Here's how the part is built. I have some questions about the finished solid (model axes, mm). Face numbers are marked on the shaded views. A direction names the side the tool comes from. Coordinates: 2 decimals unless noted, no trailing zeros. Write each loop counter-clockwise with the first axis right and the second up, starting at its lowest first coordinate (ties: lowest second). Pieces come first, ordered by that corner, then holes.
(1) Please list where these lines run through material, in increasing order: probe 1 along X at (y, z) = (1.8, 101.6); probe 2 along X at (y, z) = (1.55, 127); probe 3 along Y at (x, z) = (-7.5, 73.5).
(2) Thinking about a two-plate mould opening in Z: for the marked faces 1 and 2, which applies, released by +Z, released by -Z, zero draft, split by the parting line, or undercut?
(3) Imagine slicing it at D-D, the plane z = 127. List the corners of the cut face in (x, y) for me, plus the area to 3 significant figures.
(4) Imagine slicing it at B-B, the plane z = 50.8. List the corners of the cut face in (x, y) for me, plus the area to 3 significant figures.
(5) For pin 1 Ø10 at (x, z) = (2, 153.5) entering from +Y; pin 2 Ø1.1 at (x, y) = (-7.5, 2) entering from -Z, each with a flat end and sliding along its axis, tell me the tip position at first contact or that it passes through.
(6) Which directions (+Z, -Z, +X, -X, +Y, -Y) give clear straight access to the entire face, cutting with the end or side of a thin tool? Please do the marked faces 3 and 4.
(7) Imagine slicing it at A-A, the plane x = -19.5. List the corners of the cut face in (y, z) for me, plus the area to 3 significant figures.
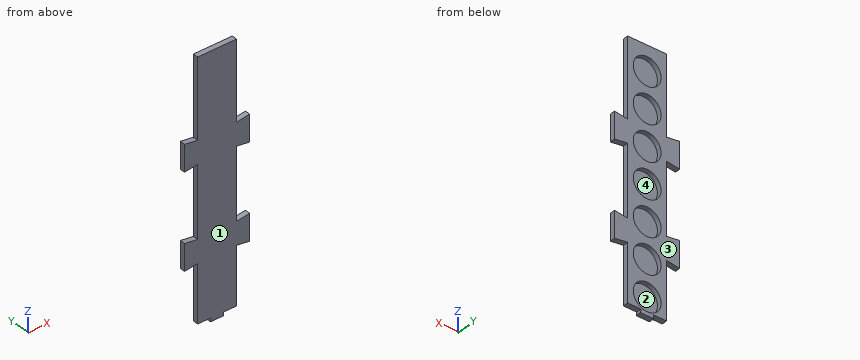
```python
from build123d import *

# Parameters (mm, degrees)
SKETCH1_W           = 27.94
SKETCH1_H           = 391.16
BOSS_EXTRUDE1_DEPTH = 3.81
SKETCH2_R           = 10
CUT_EXTRUDE1_DEPTH  = 3.21
BOSS_EXTRUDE2_DEPTH = 3.81
SKETCH7_W           = 46.80460671
SKETCH7_H           = 3.81
CUT_EXTRUDE2_DEPTH  = 210.82
BOSS_EXTRUDE4_DEPTH = 3.81


with BuildPart() as part:
    # Sketch1 → Boss-Extrude1 (new body)
    with BuildSketch(Plane(origin=(0, 0, 0), x_dir=(1, 0, 0), z_dir=(0, 1, 0))):
        Rectangle(SKETCH1_W, SKETCH1_H)
    extrude(amount=BOSS_EXTRUDE1_DEPTH)

    # Sketch2 → Cut-Extrude1 (cut)
    with BuildSketch(Plane(origin=(0, 3.81, 0), x_dir=(1, 0, 0), z_dir=(0, 1, 0))):
        with Locations(Location((0, 177.8, 0), (0, 0, 270))):
            Circle(SKETCH2_R)
        with Locations(Location((0, 152.4, 0), (0, 0, 270))):
            Circle(SKETCH2_R)
        with Locations(Location((0, 127, 0), (0, 0, 270))):
            Circle(SKETCH2_R)
        with Locations(Location((0, 101.6, 0), (0, 0, 270))):
            Circle(SKETCH2_R)
        with Locations(Location((0, 76.2, 0), (0, 0, 270))):
            Circle(SKETCH2_R)
        with Locations(Location((0, 50.8, 0), (0, 0, 270))):
            Circle(SKETCH2_R)
        with Locations(Location((0, 25.4, 0), (0, 0, 270))):
            Circle(SKETCH2_R)
        with Locations(Location((0, 0, 0), (0, 0, 270))):
            Circle(SKETCH2_R)
        with Locations(Location((0, -25.4, 0), (0, 0, 270))):
            Circle(SKETCH2_R)
        with Locations(Location((0, -50.8, 0), (0, 0, 270))):
            Circle(SKETCH2_R)
        with Locations(Location((0, -76.2, 0), (0, 0, 270))):
            Circle(SKETCH2_R)
        with Locations(Location((0, -101.6, 0), (0, 0, 270))):
            Circle(SKETCH2_R)
        with Locations(Location((0, -127, 0), (0, 0, 270))):
            Circle(SKETCH2_R)
        with Locations(Location((0, -152.4, 0), (0, 0, 270))):
            Circle(SKETCH2_R)
        with Locations(Location((0, -177.8, 0), (0, 0, 270))):
            Circle(SKETCH2_R)
    extrude(amount=-CUT_EXTRUDE1_DEPTH, mode=Mode.SUBTRACT)

    # Sketch4 → Boss-Extrude2 (add)
    with BuildSketch(Plane(origin=(0, 0, 0), x_dir=(1, 0, 0), z_dir=(0, 1, 0))):
        Polygon((23.402303355, -54.881033493), (13.97, -56.20665728), (13.97, -72.402209707), (23.402303355, -73.727833493), align=None)
        Polygon((23.402303355, 146.105623787), (13.97, 144.78), (13.97, 128.584447573), (23.402303355, 127.258823787), align=None)
        Polygon((-13.97, 128.584447573), (-13.97, 144.78), (-23.402303355, 146.105623787), (-23.402303355, 127.258823787), align=None)
        Polygon((23.402303355, 79.11007136), (13.97, 77.784447573), (13.97, 61.588895147), (23.402303355, 60.26327136), align=None)
        Polygon((23.402303355, 12.114518933), (13.97, 10.788895147), (13.97, -5.40665728), (23.402303355, -6.732281067), align=None)
        Polygon((-13.97, -5.40665728), (-13.97, 10.788895147), (-23.402303355, 12.114518933), (-23.402303355, -6.732281067), align=None)
        Polygon((-13.97, 61.588895147), (-13.97, 77.784447573), (-23.402303355, 79.11007136), (-23.402303355, 60.26327136), align=None)
        Polygon((23.402303355, -121.87658592), (13.97, -123.202209707), (13.97, -139.397762134), (23.402303355, -140.72338592), align=None)
        Polygon((-13.97, -139.397762134), (-13.97, -123.202209707), (-23.402303355, -121.87658592), (-23.402303355, -140.72338592), align=None)
        Polygon((-13.97, -72.402209707), (-13.97, -56.20665728), (-23.402303355, -54.881033493), (-23.402303355, -73.727833493), align=None)
    extrude(amount=BOSS_EXTRUDE2_DEPTH)

    # Sketch7 → Cut-Extrude2 (cut)
    with BuildSketch(Plane(origin=(0, 0, -195.58), x_dir=(-1, 0, 0), z_dir=(0, 0, -1))):
        with Locations((0, 1.905)):
            Rectangle(SKETCH7_W, SKETCH7_H)
    extrude(amount=-CUT_EXTRUDE2_DEPTH, mode=Mode.SUBTRACT)

    # Sketch8 → Boss-Extrude4 (add)
    with BuildSketch(Plane(origin=(0, 3.81, 0), x_dir=(1, 0, 0), z_dir=(0, 1, 0))):
        Polygon((-4.40552628, -15.24), (-4.7625, -12.7), (4.7625, -12.7), (4.40552628, -15.24), align=None)
    extrude(amount=-BOSS_EXTRUDE4_DEPTH)


solid = part.part
```
Recorded:
1. probe 1: x = -13.97 to -10, 10 to 13.97
1. probe 2: x = -23.4 to -10, 10 to 23.4
1. probe 3: y = 0 to 0.6
2. face 1: zero draft
2. face 2: undercut
3. outline: (-23.4, 0) - (23.4, 0) - (23.4, 3.81) - (10, 3.81) - (10, 0.6) - (-10, 0.6) - (-10, 3.81) - (-23.4, 3.81) - close
3. area: 114 mm2
4. outline: (-13.97, 0) - (13.97, 0) - (13.97, 3.81) - (10, 3.81) - (10, 0.6) - (-10, 0.6) - (-10, 3.81) - (-13.97, 3.81) - close
4. area: 42.3 mm2
5. pin 1: stops at y = 0.6
5. pin 2: stops at z = 15.24
6. face 3: +Z, -Z, +X, -X, +Y
6. face 4: +Y
7. outline: (0, 55.43) - (3.81, 55.43) - (3.81, 73.18) - (0, 73.18) - close; (0, 122.43) - (3.81, 122.43) - (3.81, 140.17) - (0, 140.17) - close
7. area: 135 mm2
